Design review of the part built by this model. Coordinates are the model's own, in mm. A direction names the side the tool comes from. Coordinates: 2 decimals unless noted, no trailing zeros. Loops run counter-clockwise (first coordinate to the right, second up) from the corner with the lowest first, then second, coordinate; pieces in that order, holes last. Notation, with made-up numbers: M 53.5,69.5 L 66.5,69.5 A22 cw 66.5,93.5 Z; hole C 56.5,13.5 d5. An arc over 180 degrees is marked long. Put each result on its own line as item: value. Start each with the question number.
(1) The part is to be moulded in two halves that separate along Y. For faces 6 (the flat face through (-18, 5.258, 4)), 7 (the cylindrical face through (-22.77, 15.61, 0.79)), 8 (the flat face through (26.226, 0, -2)), say which applies: +Y half, -Y half, draft (parallel to the pull), parting line (faces both ways), or undercut.
(2) Take a section at A-A, the plane z = -6.25. Give the boundary of the cut face in (x, y), then the cut area to 3 significant figures.
(3) For faces 1 (the flat face through (9.08, 8, 4)), 2 (the flat face through (6, 11.608, 4)), 3 (the flat face through (-9, -10, 4.775)), 4 (the flat face through (23, -3, -6.934)), 5 (the flat face through (23, 4.089, -3)), list the 3-axis set-ups (+Z, -Z, +X, -X, +Y, -Y) from which the entire face can be reached by the end or side of a thin tool; tool diameter is ignored.
(4) Take a section at D-D, the plane x = -22.5. Give the boundary of the cut face in (y, z).
(5) For probe 1 along X at (y, z) = (4, -5.75); probe 2 along Z at (x, y) = (12.5, 12); probe 3 along X at (y, z) = (-2, -9.5), list the stretches that pass through material, from the lowest coordinate up. Write a range as [from, to].
(6) Take a section at C-C, the plane y = -13.5. Give the boundary of the cut face in (x, z).
(7) Take a section at B-B, the plane z = 3.75. Give the boundary of the cut face in (x, y), then the cut area to 3 significant figures.
(8) Clearance check with flat-ended pins moving along their axes: pin 1 (3 mm diameter, centred on x = 23, z = -4, fed in from +Y); pin 2 (1.5 mm diameter, centred on x = -1.5, y = 11, fed in from +Z); pin 3 (1.2 mm diameter, centred on x = 5, z = 2.5, fed in from +Y); pin 4 (2.5 mm diameter, centred on x = -23.1, y = 14.12, fed in from -Z). State where each tip first meets the part, or that it passes through.
```python
from build123d import *

# Parameters (mm, degrees)
SKETCH1_W           = 52.451
SKETCH1_H           = 34.4932
SKETCH1_R           = 1.524
BOSS_EXTRUDE1_DEPTH = 1.6002
SKETCH2_W           = 6.35
SKETCH2_H           = 6.35
BOSS_EXTRUDE2_DEPTH = 3.937
BOSS_EXTRUDE3_DEPTH = 3.175
SKETCH4_W           = 5.7912
SKETCH4_H           = 14.986
SKETCH4_H_2         = 12.446
BOSS_EXTRUDE4_DEPTH = 6.9342
SKETCH5_W           = 5.08
SKETCH5_H           = 12.7
BOSS_EXTRUDE5_DEPTH = 11.938
SKETCH6_R           = 1.7145
BOSS_EXTRUDE6_DEPTH = 0.9144


with BuildPart() as part:
    # Sketch1 → Boss-Extrude1 (new body)
    with BuildSketch(Plane.XY):
        Rectangle(SKETCH1_W, SKETCH1_H)
        with Locations((23.1013, 14.1224)):
            Circle(SKETCH1_R, mode=Mode.SUBTRACT)
        with Locations(Location((23.1013, -14.1224, 0), (0, 0, 180))):
            Circle(SKETCH1_R, mode=Mode.SUBTRACT)
        with Locations((-23.1013, -14.1224)):
            Circle(SKETCH1_R, mode=Mode.SUBTRACT)
        with Locations(Location((-23.1013, 14.1224, 0), (0, 0, 180))):
            Circle(SKETCH1_R, mode=Mode.SUBTRACT)
    extrude(amount=BOSS_EXTRUDE1_DEPTH)

    # Sketch2 → Boss-Extrude2 (add)
    with BuildSketch(Plane.XY.offset(1.6002)):
        with Locations((-18.0975, 8.4328)):
            Rectangle(SKETCH2_W, SKETCH2_H)
        with Locations((-5.9055, 8.4328)):
            Rectangle(SKETCH2_W, SKETCH2_H)
        with Locations((18.0975, 8.4328)):
            Rectangle(SKETCH2_W, SKETCH2_H)
        with Locations((5.9055, 8.4328)):
            Rectangle(SKETCH2_W, SKETCH2_H)
    extrude(amount=BOSS_EXTRUDE2_DEPTH)

    # Sketch3 → Boss-Extrude3 (add)
    with BuildSketch(Plane.XY.offset(1.6002)):
        with BuildLine():
            Line((-12.3317, -8.6614), (-5.2197, -8.6614))
            ThreePointArc((-5.2197, -8.6614), (-4.142069265, -9.107769265), (-3.6957, -10.1854))
            Line((-3.6957, -10.1854), (-3.6957, -10.6426))
            ThreePointArc((-3.6957, -10.6426), (-4.142069265, -11.720230735), (-5.2197, -12.1666))
            Line((-5.2197, -12.1666), (-12.3317, -12.1666))
            ThreePointArc((-12.3317, -12.1666), (-13.409330735, -11.720230735), (-13.8557, -10.6426))
            Line((-13.8557, -10.6426), (-13.8557, -10.1854))
            ThreePointArc((-13.8557, -10.1854), (-13.409330735, -9.107769265), (-12.3317, -8.6614))
        make_face()
    extrude(amount=BOSS_EXTRUDE3_DEPTH)

    # Sketch4 → Boss-Extrude4 (add)
    with BuildSketch(Plane(origin=(0, 0, 0), x_dir=(-1, 0, 0), z_dir=(0, 0, -1))):
        with Locations((-23.3299, -3.4036)):
            Rectangle(SKETCH4_W, SKETCH4_H)
        with Locations((23.3299, 1.9812)):
            Rectangle(SKETCH4_W, SKETCH4_H_2)
    extrude(amount=BOSS_EXTRUDE4_DEPTH)

    # Sketch5 → Boss-Extrude5 (add)
    with BuildSketch(Plane(origin=(0, 0, 0), x_dir=(-1, 0, 0), z_dir=(0, 0, -1))):
        with Locations((9.7155, -1.0668)):
            Rectangle(SKETCH5_W, SKETCH5_H)
    extrude(amount=BOSS_EXTRUDE5_DEPTH)

    # Sketch6 → Boss-Extrude6 (add)
    with BuildSketch(Plane.XY.offset(5.5372)):
        with Locations((-18.0975, 8.4328)):
            Circle(SKETCH6_R)
        with Locations((-5.9055, 8.4328)):
            Circle(SKETCH6_R)
        with Locations((5.9055, 8.4328)):
            Circle(SKETCH6_R)
        with Locations((18.0975, 8.4328)):
            Circle(SKETCH6_R)
    extrude(amount=BOSS_EXTRUDE6_DEPTH)


solid = part.part
```
Computed values:
1. face 6: -Y half
1. face 7: undercut
1. face 8: draft
2. outline: M -26.23,-4.24 L -20.43,-4.24 L -20.43,8.2 L -26.23,8.2 Z; M -12.26,-7.42 L -7.18,-7.42 L -7.18,5.28 L -12.26,5.28 Z; M 20.43,-10.9 L 26.23,-10.9 L 26.23,4.09 L 20.43,4.09 Z
2. area: 223 mm^2
3. face 1: +Z, +Y, -Y
3. face 2: +Z, +X, -X, +Y
3. face 3: +Z, +X, -X, -Y
3. face 4: -Z, +X, +Y, -Y
3. face 5: -Z, +X, +Y
4. outline: M -17.25,0 L -15.52,0 L -15.52,1.6 L -17.25,1.6 Z; M -12.72,0 L -4.24,0 L -4.24,-6.93 L 8.2,-6.93 L 8.2,0 L 12.72,0 L 12.72,1.6 L -12.72,1.6 Z; M 15.52,0 L 17.25,0 L 17.25,1.6 L 15.52,1.6 Z
5. probe 1: x = [-26.23, -20.43], [-12.26, -7.18], [20.43, 26.23]
5. probe 2: z = [0, 1.6]
5. probe 3: x = [-12.26, -7.18]
6. outline: M -26.23,0 L -24.49,0 L -24.49,1.6 L -26.23,1.6 Z; M -21.71,0 L 21.71,0 L 21.71,1.6 L -21.71,1.6 Z; M 24.49,0 L 26.23,0 L 26.23,1.6 L 24.49,1.6 Z
7. outline: M -21.27,5.26 L -14.92,5.26 L -14.92,11.61 L -21.27,11.61 Z; M -13.86,-10.64 A1.52 ccw -12.33,-12.17 L -5.22,-12.17 A1.52 ccw -3.7,-10.64 L -3.7,-10.19 A1.52 ccw -5.22,-8.66 L -12.33,-8.66 A1.52 ccw -13.86,-10.19 Z; M -9.08,5.26 L -2.73,5.26 L -2.73,11.61 L -9.08,11.61 Z; M 2.73,5.26 L 9.08,5.26 L 9.08,11.61 L 2.73,11.61 Z; M 14.92,5.26 L 21.27,5.26 L 21.27,11.61 L 14.92,11.61 Z
7. area: 195 mm^2
8. pin 1: stops at y = 4.09
8. pin 2: stops at z = 1.6
8. pin 3: stops at y = 11.61
8. pin 4: passes through
